Source: CAD feature listing. Evaluate the final solid. Frame: model axes, mm. A direction names the side the tool comes from. Coordinates: 2 decimals unless noted, no trailing zeros. Loops run counter-clockwise (first coordinate to the right, second up) from the corner with the lowest first, then second, coordinate; pieces in that order, holes last. Notation, with made-up numbers: (42.25, -11) -> (52.25, -11) arc R26 cw to (52.25, 21) -> close; hole circle Ø6 at (-33, 60). An arc over 180 degrees is marked (long way). Answer as CSV lines item,"result".
from build123d import *

# Parameters (mm, degrees)
SKETCH053_R  = 1
PAD040_DEPTH = 7
ARRAY_COUNT  = 3
SKETCH052_R  = 6
PAD039_DEPTH = 36
SKETCH_R     = 35.5
PAD_DEPTH    = 37.5


with BuildPart() as array:
    # Sketch053 → Pad040 (new body)
    with BuildSketch(Plane.XY):
        with Locations((0, 28.4)):
            Circle(SKETCH053_R)
    extrude(amount=PAD040_DEPTH)

    # Array: Array ×3 about axis
    array_axis = Axis((0, 0, 0), (0, 0, 1))


with BuildPart() as array_1:
    add(array.part)
    for i in range(1, ARRAY_COUNT):
        add(array.part.rotate(array_axis, i * 360 / ARRAY_COUNT))


with BuildPart() as body032:
    # Sketch052 → Pad039 (new body)
    with BuildSketch(Plane.XZ):
        with Locations((-22.4, 13)):
            Circle(SKETCH052_R)
    extrude(amount=PAD039_DEPTH)


with BuildPart() as blower:
    # Sketch → Pad (new body)
    with BuildSketch(Plane.XY):
        Circle(SKETCH_R)
    extrude(amount=PAD_DEPTH)

    # Fusion: union Body032
    add(body032.part)

    # Cut: cut Array
    add(array_1.part, mode=Mode.SUBTRACT)


solid = blower.part
(1) Material intervals for L1, parallel to X at y = 28.4, z = 5; L2, parallel to Y at x = -32, z = 22.5; L3, parallel to Y at x = -24, z = 24, sorted ascending. Write a range as [from, to].
Computed values:
L1,"[-21.3, -1], [1, 21.3]"
L2,"[-15.37, 15.37]"
L3,"[-26.16, 26.16]"
(2) Cut plane A-A (y = 28.4). Return the cut outline in (x, z), then the cut area to 3 significant figures.
Computed values:
outline,"(-21.3, 0) -> (-1, 0) -> (-1, 7) -> (1, 7) -> (1, 0) -> (21.3, 0) -> (21.3, 37.5) -> (-21.3, 37.5) -> close"
area,"1,580 mm^2"
(3) Access query for faces 3 (the cylindrical face through (-25.594, -14.156, 3.451)), 4 (the cylindrical face through (-28.394, -30.18, 13.264)), 5 (the flat face through (-22, -36, 13)). Directions: +Z, -Z, +X, -X, +Y, -Y. A direction counts if a zero-diameter tool reaches every point of the face in a straight line with its end or side. Return the directions, or none.
Computed values:
face 3,"-Z"
face 4,"-Y"
face 5,"+Z, -Z, +X, -X, -Y"
(4) Cut plane D-D (z = 3). Return the cut outline in (x, y), then the cut area to 3 significant figures.
Computed values:
outline,"circle Ø71 at (0, 0); hole circle Ø2 at (-24.6, -14.2); hole circle Ø2 at (0, 28.4); hole circle Ø2 at (24.6, -14.2)"
area,"3,950 mm^2"
(5) Draft query along X for faces 1 (the flat face through (0, 0, 0)), 2 (the cylindrical face through (-0.13, 29.39, 3.45)). Return one class per face: released by +X, released by -X, zero draft, split by the parting line, or undercut.
Computed values:
face 1,"zero draft"
face 2,"undercut"
(6) Cut plane B-B (z = 28.5). Return the cut outline in (x, y), then the cut area to 3 significant figures.
Computed values:
outline,"circle Ø71 at (0, 0)"
area,"3,960 mm^2"
(7) Cut plane C-C (x = -22.4). Return the cut outline in (y, z).
Computed values:
outline,"(-36, 7) -> (-27.54, 7) -> (-27.54, 0) -> (27.54, 0) -> (27.54, 37.5) -> (-27.54, 37.5) -> (-27.54, 19) -> (-36, 19) -> close"
(8) Pin query (flat end, axial travel): pin 1 Ø6 at (y, z) = (-16.5, 33) entering from +X; pin 2 Ø10 at (x, y) = (18.5, 20.5) entering from -Z; pin 3 Ø1.2 at (x, y) = (0, 28.4) entering from -Z; pin 4 Ø3 at (y, z) = (27.5, 32) entering from -X. Return the tip coordinate at first contact, or that it passes through.
Computed values:
pin 1,"x = 32.83"
pin 2,"z = 0"
pin 3,"z = 7"
pin 4,"x = -24.17"
